```python
from build123d import *

# Parameters (mm, degrees)
SKETCH2_R           = 10
BOSS_EXTRUDE1_DEPTH = 23
SKETCH3_R           = 5
BOSS_EXTRUDE2_DEPTH = 20
BOSS_EXTRUDE3_START = 10
SKETCH4_R           = 5
BOSS_EXTRUDE3_DEPTH = 10
CHAMFER1_SIZE       = 1
CHAMFER2_SIZE       = 1


with BuildPart() as part:
    # Sketch2 → Boss-Extrude1 (new body)
    with BuildSketch(Plane.XY):
        Circle(SKETCH2_R)
    extrude(amount=BOSS_EXTRUDE1_DEPTH)

    # Sketch3 → Boss-Extrude2 (add)
    with BuildSketch(Plane.XY.offset(23)):
        Circle(SKETCH3_R)
    extrude(amount=BOSS_EXTRUDE2_DEPTH)

    # Sketch4 → Boss-Extrude3 (add)
    with BuildSketch(Plane(origin=(0, 0, 0), x_dir=(-1, 0, 0), z_dir=(0, 0, -1)).offset(BOSS_EXTRUDE3_START)):
        with Locations(Location((0, 0, 0), (0, 0, 180))):
            Circle(SKETCH4_R)
    extrude(amount=-BOSS_EXTRUDE3_DEPTH)

    # Chamfer1
    chamfer1_edges = [part.edges().sort_by_distance(p)[0] for p in [
        (-5, 0, -10),
    ]]
    chamfer(chamfer1_edges, length=CHAMFER1_SIZE)

    # Chamfer2
    chamfer2_edges = [part.edges().sort_by_distance(p)[0] for p in [
        (-5, 0, 43),
    ]]
    chamfer(chamfer2_edges, length=CHAMFER2_SIZE)


solid = part.part
```
Here's how the part is built. I have some questions about the finished solid (model axes, mm). A direction names the side the tool comes from. Give positions to 0.01 mm unless a question says otherwise; leave off trailing zeros. Loops run counter-clockwise (first coordinate to the right, second up) from the corner with the lowest first, then second, coordinate; pieces in that order, holes last. Notation, with made-up numbers: M 30,48.25 L 37,48.25 A29 ccw 37,83.25 Z; hole C -37,51.5 d10. An arc over 180 degrees is marked long. Put each result on its own line as item: value. Start each with the question number.
(1) If we mould it in two halves opening along Y, with no side actions, what happens to faces 4 (the cylindrical face through (-2.17, -9.76, 11.34)), 5 (the flat face through (-5, -2, 0))? For each: +Y half, -Y half, draft (parallel to the pull), parting line (faces both ways), or undercut.
(2) I want a section at C-C on z = -0.5. Please give me the cut outline in (x, y), then the cut area to 3 significant figures.
(3) For faces 1 (the flat face through (0, 0, -10)), 2 (the cylindrical face through (-1.08, -4.88, 32.37)), 3 (the cylindrical face through (-5, 0, -5)), which set-ups out of +Z, -Z, +X, -X, +Y, -Y let a thin tool reach every point of the face, with its end or its side?
(4) I want a section at A-A on x = 0. Please give me the cut outline in (y, z).
(5) I want a section at D-D on y = -8. Please give me the cut outline in (x, z), then the cut area to 3 significant figures.
(6) Will these pins go through, and if not, where does the flat tip stop? pin 1 Ø5 at (y, z) = (7.5, 16.5) entering from -X; pin 2 Ø2 at (x, z) = (3, 17.5) entering from -Y; pin 3 Ø4 at (x, y) = (-5.5, 4.5) entering from +Z.
(7) I need wall thicknesses on line 1 along Z through (x, y) = (-5.25, -7); line 2 along X through (y, z) = (-0.25, 10.5); line 3 along Y through (x, z) = (0.25, 25). Which ranges of each line are inside material? Lowest first, please. Write a range as [from, to].
Answer block:
1. face 4: parting line
1. face 5: draft
2. outline: C 0,0 d10
2. area: 78.5 mm^2
3. face 1: -Z, +X, -X, +Y, -Y
3. face 2: +Z
3. face 3: -Z
4. outline: M -10,0 L -5,0 L -5,-9 L -4,-10 L 4,-10 L 5,-9 L 5,0 L 10,0 L 10,23 L 5,23 L 5,42 L 4,43 L -4,43 L -5,42 L -5,23 L -10,23 Z
5. outline: M -6,0 L 6,0 L 6,23 L -6,23 Z
5. area: 276 mm^2
6. pin 1: x = -8.66
6. pin 2: y = -9.8
6. pin 3: z = 23
7. line 1: [0, 23]
7. line 2: [-10, 10]
7. line 3: [-4.99, 4.99]
